Geometry: final body of the model. Coordinates: model frame, mm. Give positions to 0.01 mm unless a question says otherwise; leave off trailing zeros. Order: outer loops, then holes, each group sorted by start corner. A loop starts at its lowest first (then second) coordinate and runs counter-clockwise, first axis right, second up. Notation, with made-up numbers: M 34.25,66 L 92.25,66 A16 cw 92.25,76 Z; hole C 19,48.5 d9. An arc over 180 degrees is marked long. Use CSV: the item, a comma, the result in double quotes.
```python
from build123d import *

# Parameters (mm, degrees)
SKETCH1_W                 = 12.7
SKETCH1_H                 = 12.7
BOSS_EXTRUDE1_DEPTH       = 2.54
F_4_CLEARANCE_HOLE1_D     = 3.2639
TAP_DRILL_FOR_4_40_TAP1_D = 2.2606


with BuildPart() as part:
    # Sketch1 → Boss-Extrude1 (new body)
    with BuildSketch(Plane(origin=(0, 0, 0), x_dir=(1, 0, 0), z_dir=(0, 1, 0))):
        Rectangle(SKETCH1_W, SKETCH1_H)
    extrude(amount=BOSS_EXTRUDE1_DEPTH)

    # #4 Clearance Hole1 (through all)
    with Locations(Plane(origin=(0, 2.54, -2.54), x_dir=(0, 0, 1), z_dir=(0, 1, 0))):
        with Locations((0, 0)):
            Hole(F_4_CLEARANCE_HOLE1_D / 2)

    # Tap Drill for #4-40 Tap1 (through all)
    with Locations(Plane(origin=(0, 2.54, 2.54), x_dir=(0, 0, 1), z_dir=(0, 1, 0))):
        with Locations((0, 0)):
            Hole(TAP_DRILL_FOR_4_40_TAP1_D / 2)


solid = part.part
```
1. Section D-D, the plane z = 2.54. Return the cut outline in (x, y), plus the area to 3 significant figures.
Answer:
outline,"M -6.35,0 L -1.13,0 L -1.13,2.54 L -6.35,2.54 Z; M 1.13,0 L 6.35,0 L 6.35,2.54 L 1.13,2.54 Z"
area,"26.5 mm2"
2. Pin query (flat end, axial travel): pin 1 Ø2.5 at (x, z) = (0, -2.54) entering from -Y. Return the tip coordinate at first contact, or that it passes through.
Answer:
pin 1,"through"
3. Pull-direction query (Z, two-part tool) for faces 1 (the face through (-6.35, 1, 0)), 2 (the face through (-0.625, 1.252, -4.048)), 3 (the face through (0, 1, -6.35)); classes: +Z half, -Z half, draft (parallel to the pull), parting line (faces both ways), or undercut.
Answer:
face 1,"draft"
face 2,"undercut"
face 3,"-Z half"
4. Section C-C, the plane y = 0.6. Return the cut outline in (x, z).
Answer:
outline,"M -6.35,-6.35 L 6.35,-6.35 L 6.35,6.35 L -6.35,6.35 Z; hole C 0,-2.54 d3.26; hole C 0,2.54 d2.26"
5. Section A-A, the plane x = 0. Return the cut outline in (y, z), plus the area to 3 significant figures.
Answer:
outline,"M 0,-6.35 L 2.54,-6.35 L 2.54,-4.17 L 0,-4.17 Z; M 0,-0.91 L 2.54,-0.91 L 2.54,1.41 L 0,1.41 Z; M 0,3.67 L 2.54,3.67 L 2.54,6.35 L 0,6.35 Z"
area,"18.2 mm2"
6. Line query: line 1 (X direction, y = 1.45, z = 2.54); line 2 (X direction, y = 2, z = -2.54). Output: solid intervals per line, ascending.
Answer:
line 1,"-6.35 to -1.13, 1.13 to 6.35"
line 2,"-6.35 to -1.63, 1.63 to 6.35"
7. Section B-B, the plane z = -2.54. Return the cut outline in (x, y).
Answer:
outline,"M -6.35,0 L -1.63,0 L -1.63,2.54 L -6.35,2.54 Z; M 1.63,0 L 6.35,0 L 6.35,2.54 L 1.63,2.54 Z"
